Autodesk Inventor part; units mm, degrees
ref_plane "YZ Plane" through (0, 0, 0) normal (1, 0, 0) x (0, 1, 0)
ref_plane "XZ Plane" through (0, 0, 0) normal (0, 1, 0) x (-1, 0, 0)
ref_plane "XY Plane" through (0, 0, 0) normal (0, 0, 1) x (1, 0, 0)
sketch "Boceto1" plane through (0, 0, 0) normal (0, 1, 0) x (-1, 0, 0)
  line L0 (30.1625, 61.9125) -> (-30.1625, 61.9125) construction
  line L1 (-30.1625, 61.9125) -> (-30.1625, -61.9125) construction
  line L2 (-30.1625, -61.9125) -> (30.1625, -61.9125) construction
  line L3 (30.1625, -61.9125) -> (30.1625, 61.9125) construction
  line L4 (30.1625, 61.9125) -> (-30.1625, -61.9125) construction
  line L5 (-30.1625, 61.9125) -> (30.1625, -61.9125) construction
  arc A0 (-34.925, -61.9125) -> (-30.1625, -66.675) centre (-30.1625, -61.9125) ccw
  arc A1 (-30.1625, 66.675) -> (-34.925, 61.9125) centre (-30.1625, 61.9125) ccw
  arc A2 (34.925, 61.9125) -> (30.1625, 66.675) centre (30.1625, 61.9125) ccw
  line L6 (34.925, -61.9125) -> (34.925, 61.9125)
  line L7 (30.1625, 66.675) -> (-30.1625, 66.675)
  line L8 (-34.925, 61.9125) -> (-34.925, -61.9125)
  line L9 (30.1625, -66.675) -> (-30.1625, -66.675)
  arc A3 (30.1625, -66.675) -> (34.925, -61.9125) centre (30.1625, -61.9125) ccw
  arc A4 (30.1625, -57.15) -> (28.0767, -57.6311) centre (30.1625, -61.9125) ccw
  point P0 (0, 0)
  dimension "d0" = 60.325
  dimension "d1" = 123.825
  dimension "d3" = 9.525
  dimension "d4" = 9.525
  dimension "d5" = 9.525
  dimension "d6" = 69.85
  dimension "d7" = 133.35
extrude "Extrusión1" add sketch "Boceto1" along normal blind 38.1
sketch "Boceto3" plane through (0, 38.1, 0) normal (0, 1, 0) x (1, 0, 0)
  line L0 (-25.4, 60.325) -> (25.4, 60.325)
  line L1 (28.575, 57.15) -> (28.575, -19.05)
  line L2 (25.4, -22.225) -> (-6.35, -22.225)
  line L3 (-9.525, -25.4) -> (-9.525, -34.925)
  line L4 (-28.575, 57.15) -> (-28.575, -34.925)
  line L5 (-25.4, -38.1) -> (-12.7, -38.1)
  line L6 (30.1625, 66.675) -> (-30.1625, 66.675)
  line L7 (-34.925, 61.9125) -> (-34.925, -61.9125)
  line L8 (34.925, -61.9125) -> (34.925, 61.9125)
  line L9 (-30.1625, -66.675) -> (30.1625, -66.675)
  arc A0 (-25.4, 60.325) -> (-28.575, 57.15) centre (-25.4, 57.15) ccw
  arc A1 (28.575, 57.15) -> (25.4, 60.325) centre (25.4, 57.15) ccw
  arc A2 (25.4, -22.225) -> (28.575, -19.05) centre (25.4, -19.05) ccw
  arc A3 (-6.35, -22.225) -> (-9.525, -25.4) centre (-6.35, -25.4) ccw
  arc A4 (-12.7, -38.1) -> (-9.525, -34.925) centre (-12.7, -34.925) ccw
  arc A5 (-28.575, -34.925) -> (-25.4, -38.1) centre (-25.4, -34.925) ccw
  point P0 (0, 0)
  dimension "d20" = 6.35
  dimension "d21" = 6.35
  dimension "d22" = 6.35
  dimension "d23" = 44.45
  dimension "d24" = 15.875
  dimension "d25" = 38.1
  dimension "d26" = 3.175
extrude "Extrusión2" cut sketch "Boceto3" against normal blind 31.75
sketch "Boceto4" plane through (-34.925, 0, -61.9125) normal (-1, 0, 0) x (0, 0, 1)
  line L0 (11.1125, 38.1) -> (71.4166, 38.1)
  line L1 (71.4166, 38.1) -> (71.4166, 20.6375)
  line L2 (69.8291, 19.05) -> (11.1125, 19.05)
  line L3 (11.1125, 19.05) -> (11.1125, 38.1)
  line L4 (-4.7625, 0) -> (-4.7625, 38.1)
  line L5 (0, 38.1) -> (123.825, 38.1)
  arc A0 (69.8291, 19.05) -> (71.4166, 20.6375) centre (69.8291, 20.6375) ccw
  point P0 (61.9125, 0)
  dimension "d29" = 15.875
  dimension "d30" = 19.05
  dimension "d31" = 60.325
  dimension "d32" = 3.175
extrude "Extrusión3" cut sketch "Boceto4" against normal blind 6.35
sketch "Boceto6" plane through (0, 0, 0) normal (0, -1, 0) x (1, 0, 0)
  circle A0 centre (-12.7, -6.35) radius 9.525
  line L0 (30.1625, -66.675) -> (-30.1625, -66.675)
  line L1 (-34.925, -61.9125) -> (-34.925, 61.9125)
  point P0 (0, 0)
  dimension "d44" = 19.05
  dimension "d45" = 60.325
  dimension "d46" = 22.225
extrude "Extrusión5" add sketch "Boceto6" against normal blind 38.1
sketch "Boceto7" plane through (0, 0, 0) normal (0, -1, 0) x (1, 0, 0)
  circle A0 centre (-12.7, -6.35) radius 9.525 construction
  line L0 (28.575, -57.15) -> (28.575, 19.05) construction
  arc A1 (28.575, 19.05) -> (25.4, 22.225) centre (25.4, 19.05) ccw construction
  line L1 (25.4, 22.225) -> (-6.35, 22.225) construction
  line L2 (-9.525, 25.4) -> (-9.525, 34.925) construction
  arc A2 (-9.525, 25.4) -> (-6.35, 22.225) centre (-6.35, 25.4) ccw construction
  arc A3 (-9.525, 34.925) -> (-12.7, 38.1) centre (-12.7, 34.925) ccw construction
  line L3 (-12.7, 38.1) -> (-25.4, 38.1) construction
  arc A4 (-25.4, 38.1) -> (-28.575, 34.925) centre (-25.4, 34.925) ccw construction
  line L4 (-28.575, 34.925) -> (-28.575, -57.15) construction
  line L5 (-25.4, -60.325) -> (25.4, -60.325) construction
  arc A5 (25.4, -60.325) -> (28.575, -57.15) centre (25.4, -57.15) ccw construction
  arc A6 (-28.575, -57.15) -> (-25.4, -60.325) centre (-25.4, -57.15) ccw construction
  point P0 (0, 0)
properties part number "Lab8A01209499P1"
The listing builds one solid part. Answer for the finished solid, in the listing's coordinates (mm). A direction names the side the tool comes from. Give positions to 0.01 mm unless a question says otherwise; leave off trailing zeros. Write each loop counter-clockwise with the first axis right and the second up, starting at its lowest first coordinate (ties: lowest second). Pieces come first, ordered by that corner, then holes. Notation, with made-up numbers: (-3, 45.5) -> (11, 45.5) arc R16 cw to (11, 54.5) -> close; hole circle Ø6 at (28.5, 7.25). An arc over 180 degrees is marked (long way). One line per question, with ' | ' between items. Start each with the question number.
1. Given pin 1 Ø1.5 at (x, z) = (17, -32) entering from +Y; pin 2 Ø7 at (x, z) = (-31.5, -35) entering from +Y; pin 3 Ø1 at (y, z) = (25.5, -28.5) entering from -X (3 decimals), each flat-ended and moving along its own axis, determine where each tip first touches the part or whether it passes through.
2. Section D-D (x = 17) is taken. Determine the outline of the cut face in (y, z) (3 decimals), plus the area to 3 significant figures.
3. Section C-C (z = -6.35) is taken. Determine the outline of the cut face in (x, y) (3 decimals).
4. For faces 1 (the flat face through (-32, 28, -50.8)), 2 (the flat face through (8, 38.1, 31)), 3 (the cylindrical face through (27.67, 22.45, -59.37)), determine the directions among +Z, -Z, +X, -X, +Y, -Y from which every point of the face is accessible in a straight line to the end or side of a thin tool.
5. Find the intervals of material crossed by probe 1 along Z at (x, y) = (5, 22) (3 decimals); probe 2 along Z at (x, y) = (-19.5, 8.5) (3 decimals); probe 3 along X at (y, z) = (36, 27.5) (3 decimals), in increasing order.
6. Section A-A (y = 15) is taken. State how many separate pieces and enclosed holes the cut face has, plus the area to 3 significant figures.
Response values:
1) pin 1: y = 6.35 | pin 2: y = 19.05 | pin 3: x = 28.575
2) outline: (0, -66.675) -> (38.1, -66.675) -> (38.1, -60.325) -> (6.35, -60.325) -> (6.35, 22.225) -> (38.1, 22.225) -> (38.1, 66.675) -> (0, 66.675) -> close | area: 2,460 mm2
3) outline: (-34.925, 0) -> (34.925, 0) -> (34.925, 38.1) -> (28.575, 38.1) -> (28.575, 6.35) -> (-3.175, 6.35) -> (-3.175, 38.1) -> (-22.225, 38.1) -> (-22.225, 6.35) -> (-28.575, 6.35) -> (-28.575, 19.05) -> (-34.925, 19.05) -> close
4) face 1: -X, +Y | face 2: +Z, -Z, +X, -X, +Y | face 3: +Y
5) probe 1: -66.675 to -60.325, 22.225 to 66.675 | probe 2: -66.675 to -60.325, -13.02 to 0.32, 38.1 to 66.675 | probe 3: -34.925 to -28.575, -9.525 to 34.925
6) separate pieces: 2 | enclosed holes: 1 | area: 4,570 mm2
